Geometry: final body of the model. Coordinates: model frame, mm. A direction names the side the tool comes from. Coordinates: 2 decimals unless noted, no trailing zeros. Write each loop counter-clockwise with the first axis right and the second up, starting at its lowest first coordinate (ties: lowest second). Pieces come first, ordered by that corner, then holes. Notation, with made-up numbers: (-36.5, 24) -> (1.5, 24) arc R25 cw to (1.5, 47) -> close; hole circle Ø1 at (60.25, -9.75). An arc over 180 degrees is marked (long way). One line per item, written item: value.
Autodesk Inventor part; units mm, degrees
ref_plane "YZ Plane" through (0, 0, 0) normal (1, 0, 0) x (0, 1, 0)
ref_plane "XZ Plane" through (0, 0, 0) normal (0, 1, 0) x (-1, 0, 0)
ref_plane "XY Plane" through (0, 0, 0) normal (0, 0, 1) x (1, 0, 0)
sketch "Sketch1" plane through (0, 0, 0) normal (1, 0, 0) x (0, 1, 0)
  line L0 (0, 0) -> (63, 0)
  line L1 (63, 0) -> (63, -113)
  line L2 (63, -113) -> (0, -113)
  line L3 (0, -113) -> (0, 0)
  line L4 (0, 0) -> (-1.5, 0)
  line L5 (-1.5, 0) -> (-1.5, 1.5)
  line L6 (-1.5, 1.5) -> (64.5, 1.5)
  line L7 (64.5, 1.5) -> (64.5, -114.5)
  line L8 (64.5, -114.5) -> (-1.5, -114.5)
  line L9 (-1.5, -114.5) -> (-1.5, 1.5)
  dimension "d0" = 63
  dimension "d1" = 113
  dimension "d2" = 1.5
  dimension "d3" = 1.5
  dimension "d4" = 66
  dimension "d5" = 116
extrude "Extrusion1" add sketch "Sketch1" along normal blind 47
sketch "Sketch2" plane through (47, 0, 0) normal (1, 0, 0) x (0, 0, -1)
  line L0 (114.5, -1.5) -> (114.5, 64.5)
  line L1 (114.5, 64.5) -> (-1.5, 64.5)
  line L2 (-1.5, 64.5) -> (-1.5, -1.5)
  line L3 (-1.5, -1.5) -> (114.5, -1.5)
  line L4 (0, 0) -> (0, 63)
  line L5 (0, 63) -> (113, 63)
  line L6 (113, 63) -> (113, 0)
  line L7 (113, 0) -> (0, 0)
extrude "Extrusion2" add sketch "Sketch2" along normal blind 1.5 contours L3 L2 L1 L0 | L4 L5 L6 L7
sketch "Sketch3" plane through (0, -1.5, 1.5) normal (0, 0, 1) x (1, 0, 0)
  line L0 (0, 66) -> (0, 0)
  line L1 (0, 0) -> (48.5, 0)
  line L2 (48.5, 66) -> (48.5, 0)
  line L3 (0, 66) -> (48.5, 66)
  line L4 (0, 0) -> (0, 66)
  line L5 (0, 66) -> (0, 33)
  line L6 (0, 33) -> (0, 13)
  line L7 (0, 13) -> (30, 13)
  line L8 (30, 13) -> (30, 53)
  line L9 (30, 53) -> (0, 53)
  point P0 (0, 1.5)
  dimension "d10" = 33
  dimension "d11" = 20
  dimension "d12" = 30
  dimension "d13" = 90
  dimension "d14" = 40
extrude "Extrusion3" cut sketch "Sketch3" against normal blind 1.5 contours L9 L8 L7 L0
sketch "Sketch4" plane through (0, -1.5, -114.5) normal (0, 0, -1) x (-1, 0, 0)
  line L0 (0, 0) -> (0, 66)
  line L1 (0, 66) -> (-48.5, 66)
  line L2 (-48.5, 0) -> (-48.5, 66)
  line L3 (0, 0) -> (-48.5, 0)
  line L4 (0, 0) -> (-48.5, 0)
  line L5 (0, 0) -> (0, 33)
  line L6 (0, 33) -> (0, 40.5)
  line L7 (0, 40.5) -> (-20, 40.5)
  line L8 (-20, 40.5) -> (-20, 25.5)
  line L9 (-20, 25.5) -> (0, 25.5)
  line L10 (0, 64.5) -> (0, 1.5)
  line L11 (0, 33) -> (0, 25.5)
  dimension "d17" = 33
  dimension "d18" = 7.5
  dimension "d19" = 20
  dimension "d20" = 15
extrude "Extrusion4" cut sketch "Sketch4" against normal blind 1.5 contours L9 L8 L7 L0
fillet "Fillet1" radius 0.5 8 edges at (24.25, -1.5, -114.5) (48.5, 31.5, -114.5) (48.5, -1.5, -56.5) (48.5, 31.5, 1.5) (24.25, -1.5, 1.5) (24.25, 64.5, -114.5) (48.5, 64.5, -56.5) (24.25, 64.5, 1.5)
properties part number "carcasa_exterior"
(1) First-contact query: pin 1 (19 mm diameter, centred on y = 30, z = -38, fed in from -X); pin 2 (1.2 mm diameter, centred on y = 22.5, z = 0.5, fed in from -X); pin 3 (1.6 mm diameter, centred on y = 33, z = -114, fed in from -X). Flat tips, straight axial feed; report the tip coordinate or a pass-through.
Responses:
pin 1: stops at x = 47
pin 2: stops at x = 30
pin 3: stops at x = 20
(2) Section C-C (y = 40.5). Return the cut outline in (x, z), then the cut area to 3 significant figures.
Responses:
outline: (0, -114.5) -> (48, -114.5) arc R0.5 ccw to (48.5, -114) -> (48.5, 1) arc R0.5 ccw to (48, 1.5) -> (30, 1.5) -> (30, 0) -> (47, 0) -> (47, -113) -> (0, -113) -> close
area: 270 mm2
(3) Line query: line 1 (Y direction, x = 17, z = -20.5); line 2 (Z direction, x = 34, y = 27.5); line 3 (X direction, y = 16, z = -103). Output: solid intervals per line, ascending. Write a range as [from, to].
Responses:
line 1: y = [-1.5, 0], [63, 64.5]
line 2: z = [-114.5, -113], [0, 1.5]
line 3: x = [47, 48.5]
(4) Section A-A (x = 36.5). Return the cut outline in (y, z), then the cut area to 3 significant figures.
Responses:
outline: (-1.5, -114) arc R0.5 ccw to (-1, -114.5) -> (64, -114.5) arc R0.5 ccw to (64.5, -114) -> (64.5, 1) arc R0.5 ccw to (64, 1.5) -> (-1, 1.5) arc R0.5 ccw to (-1.5, 1) -> close; hole (0, -113) -> (63, -113) -> (63, 0) -> (0, 0) -> close
area: 537 mm2
(5) Section D-D (x = 28). Return the cut outline in (y, z), then the cut area to 3 significant figures.
Responses:
outline: (-1.5, -114) arc R0.5 ccw to (-1, -114.5) -> (64, -114.5) arc R0.5 ccw to (64.5, -114) -> (64.5, 1) arc R0.5 ccw to (64, 1.5) -> (51.5, 1.5) -> (51.5, 0) -> (63, 0) -> (63, -113) -> (0, -113) -> (0, 0) -> (11.5, 0) -> (11.5, 1.5) -> (-1, 1.5) arc R0.5 ccw to (-1.5, 1) -> close
area: 477 mm2
(6) Reachability of faces 5 (the flat face through (23, 63, -56)), 6 (the flat face through (24, -1.5, -57)) from +Z, -Z, +X, -X, +Y, -Y: full face, straight path, thin tool, end or side. Return the list, or none.
Responses:
face 5: -X
face 6: +Z, -Z, +X, -X, -Y
(7) Section B-B (x = 11.5). Return the cut outline in (y, z), then the cut area to 3 significant figures.
Responses:
outline: (-1.5, -114) arc R0.5 ccw to (-1, -114.5) -> (24, -114.5) -> (24, -113) -> (0, -113) -> (0, 0) -> (11.5, 0) -> (11.5, 1.5) -> (-1, 1.5) arc R0.5 ccw to (-1.5, 1) -> close; (39, -114.5) -> (64, -114.5) arc R0.5 ccw to (64.5, -114) -> (64.5, 1) arc R0.5 ccw to (64, 1.5) -> (51.5, 1.5) -> (51.5, 0) -> (63, 0) -> (63, -113) -> (39, -113) -> close
area: 454 mm2
(8) Pull-direction query (Z, two-part tool) for faces 1 (the flat face through (34, 31, 1.5)), 2 (the flat face through (23, 0, -57)), 3 (the flat face through (0, -1, -56)), 4 (the flat face through (24, 32, -114.5)); classes: released by +Z, released by -Z, zero draft, split by the parting line, or undercut.
Responses:
face 1: released by +Z
face 2: undercut
face 3: zero draft
face 4: released by -Z
